from build123d import *

# Parameters (mm, degrees)
F0_W          = 5.842
F0_H          = 12.7
F0_R          = 3.175
F2_DEPTH      = 3.175
F4_R          = 1.524
F5_DEPTH      = 7.62
F5_DEPTH_BACK = 1.27
F6_R          = 1.524
F7_DEPTH      = 9.69487
F8_R          = 1.524
F9_DEPTH      = 6.87652


with BuildPart() as f1:
    # F0 (on Front) → F1 (revolve)
    with BuildSketch(Plane.XZ):
        Polygon((5.842, 12.7), (5.842, 0), (66.294, 0), (66.294, 12.7), (56.134, 12.7), (56.134, 10.16), (10.16, 10.16), (10.16, 12.7), align=None)
        with Locations((2.921, 6.35)):
            Rectangle(F0_W, F0_H)
    revolve(axis=Axis((33.147, 0, 0), (-1, 0, 0)))

    # F0 (on Front) → F2 (join, symmetric)
    with BuildSketch(Plane.XZ):
        with BuildLine():
            Line((-0.9398, 0), (0, 0))
            Line((0, 0), (0, 12.7))
            Line((0, 12.7), (5.842, 12.7))
            Line((5.842, 12.7), (5.842, 15.24))
            Line((5.842, 15.24), (-0.508, 15.24))
            Line((-0.508, 15.24), (-10.88063, 3.847543))
            ThreePointArc((-10.88063, 3.847543), (-4.591961, 5.329721), (-0.9398, 0))
        make_face()
        with BuildLine():
            ThreePointArc((-8.182663, -5.506983), (-3.195791, -4.549339), (-0.9398, 0))
            ThreePointArc((-0.9398, 0), (-4.591961, 5.329721), (-10.88063, 3.847543))
            ThreePointArc((-10.88063, 3.847543), (-12.145978, -1.583727), (-8.182663, -5.506983))
        make_face()
        with Locations((-6.6548, 0)):
            Circle(F0_R, mode=Mode.SUBTRACT)
        with BuildLine():
            Line((5.842, 0), (0, 0))
            Line((0, 0), (-0.9398, 0))
            ThreePointArc((-0.9398, 0), (-3.195791, -4.549339), (-8.182663, -5.506983))
            Line((-8.182663, -5.506983), (5.842, -9.398))
            Line((5.842, -9.398), (5.842, 0))
        make_face()
        with Locations((2.921, 6.35)):
            Rectangle(F0_W, F0_H)
    extrude(amount=F2_DEPTH, both=True)

    # F4 (on face) → F5 (join, two sides)
    with BuildSketch(Plane.YZ.offset(66.294)) as f5_sk:
        with BuildLine():
            ThreePointArc((-5.076443, 0), (0.003557, -5.08), (5.083557, 0))
            ThreePointArc((5.083557, 0), (5.083354, 0.045348), (5.082747, 0.090693))
            ThreePointArc((5.082747, 0.090693), (-0.041792, 5.079798), (-5.076443, 0))
        make_face()
        with Locations((0.003557, 0)):
            Circle(F4_R, mode=Mode.SUBTRACT)
        with BuildLine():
            ThreePointArc((-5.076443, 0), (-0.041792, 5.079798), (5.082747, 0.090693))
            Line((5.082747, 0.090693), (4.812307, 15.236546))
            Line((4.812307, 15.236546), (-5.076443, 15.186192))
            Line((-5.076443, 15.186192), (-5.076443, 0))
        make_face()
    extrude(amount=F5_DEPTH)
    extrude(f5_sk.sketch, amount=-F5_DEPTH_BACK)

    # F6 (on face) → F7 (join)
    with BuildSketch(Plane(origin=(0, -0.077459, 15.211647), x_dir=(1, 0, 0), z_dir=(0, -0.005092, 0.999987))):
        with Locations((69.043599, -0.720831)):
            Circle(F6_R)
    extrude(amount=-F7_DEPTH)

    # F8 (on face) → F9 (join)
    with BuildSketch(Plane(origin=(0, -0.077459, 15.211647), x_dir=(1, 0, 0), z_dir=(0, -0.005092, 0.999987))):
        with Locations((69.499604, 0.040541)):
            Circle(F8_R)
    extrude(amount=-F9_DEPTH)


solid = f1.part
Source: CAD feature listing. Evaluate the final solid. Frame: model axes, mm. A direction names the side the tool comes from. Coordinates: 2 decimals unless noted, no trailing zeros. Loops run counter-clockwise (first coordinate to the right, second up) from the corner with the lowest first, then second, coordinate; pieces in that order, holes last. Notation, with made-up numbers: (72, 27.5) -> (117, 27.5) arc R24 ccw to (117, 60.5) -> close; hole circle Ø5 at (42, 33). An arc over 180 degrees is marked (long way). Answer in a Markdown table with one row per item. Add a question column.
Q1. Contact query for flat-ended pins moving along their axis: pin 1 Ø1 at (x, z) = (62.5, 4.5) entering from -Y; pin 2 Ø1.5 at (x, z) = (1, 8) entering from +Y; pin 3 Ø8 at (x, z) = (18, 8.5) entering from -Y. Output: stop coordinate, or through.
Q2. Section B-B on x = 32. Return the cut outline in (y, z), and give its area (3 significant figures).
Q3. Reachability of faces 1 (the face through (10.16, 9, 6)), 2 (the face through (66.294, 0, 0)), 3 (the face through (0, -5, 0)), 4 (the face through (70.05, -0.11, -5.08)) from +Z, -Z, +X, -X, +Y, -Y: full face, straight path, thin tool, end or side. Return the list, or none.
Q4. Pull-direction query (Z, two-part tool) for faces 5 (the face through (-4.149, -0.044, -6.626)), 6 (the face through (-3.626, 0.044, 0.954)), 7 (the face through (73.914, 0, 5)); classes: pulls with the +Z half, pulls with the -Z half, needs draft (parallel to the pull), parting line crosses it, or undercut.
Q5. Section C-C on y = 6.75. Return the cut outline in (x, z), and give its area (3 significant figures).
Q6. Ray query, line 1 along X through (y, z) = (4.5, -11); line 2 along Z through (x, y) = (24, 0.25); line 3 along X through (y, z) = (5.5, -2.5). Return the intervals inside material, ascending.
Q7. Section A-A on z = 6.25. Return the cut outline in (x, y) (3 decimals), and give its area (3 significant figures).
Computed values:
| question | item | result |
|---|---|---|
| 1 | pin 1 | stops at y = -12.05 |
| 1 | pin 2 | stops at y = 10.43 |
| 1 | pin 3 | stops at y = -9.11 |
| 2 | outline | circle Ø20.32 at (0, 0) |
| 2 | area | 324 mm^2 |
| 3 | face 1 | none |
| 3 | face 2 | +X |
| 3 | face 3 | -Z, -X |
| 3 | face 4 | -Z, +X |
| 4 | face 5 | pulls with the -Z half |
| 4 | face 6 | undercut |
| 4 | face 7 | needs draft |
| 5 | outline | (0, -10.76) -> (10.16, -10.76) -> (10.16, -7.59) -> (56.13, -7.59) -> (56.13, -10.76) -> (66.29, -10.76) -> (66.29, 10.76) -> (56.13, 10.76) -> (56.13, 7.59) -> (10.16, 7.59) -> (10.16, 10.76) -> (0, 10.76) -> close |
| 5 | area | 1,140 mm^2 |
| 6 | line 1 | x = 0 to 10.16, 56.13 to 66.29 |
| 6 | line 2 | z = -10.16 to 10.16 |
| 6 | line 3 | x = 0 to 66.29 |
| 7 | outline | (-8.693, -3.175) -> (0, -3.175) -> (0, -11.056) -> (10.16, -11.056) -> (10.16, -8.01) -> (56.134, -8.01) -> (56.134, -11.056) -> (66.294, -11.056) -> (66.294, -5.076) -> (73.914, -5.076) -> (73.914, 4.973) -> (66.294, 4.973) -> (66.294, 11.056) -> (56.134, 11.056) -> (56.134, 8.01) -> (10.16, 8.01) -> (10.16, 11.056) -> (0, 11.056) -> (0, 3.175) -> (-8.693, 3.175) -> close |
| 7 | area | 1,320 mm^2 |
